from build123d import *

# Parameters (mm, degrees)
F0_R     = 25.4
F0_R_2   = 24.13
F1_DEPTH = 57.15
F3_DEPTH = 50.8


with BuildPart() as f1:
    # F0 (on Right) → F1 (new body, symmetric)
    with BuildSketch(Plane.YZ):
        with Locations((0, -25.4)):
            Circle(F0_R)
        with Locations((0, -25.4)):
            Circle(F0_R_2, mode=Mode.SUBTRACT)
    extrude(amount=F1_DEPTH, both=True)

    # F2 (on Top) → F3 (cut)
    with BuildSketch(Plane.XY):
        with BuildLine():
            ThreePointArc((48.895, -19.05), (47.9650640303, -16.8049359697), (45.72, -15.875))
            ThreePointArc((45.72, -15.875), (43.4749359697, -21.2950640303), (48.895, -19.05))
        make_face()
        with BuildLine():
            ThreePointArc((-42.545, -19.05), (-43.4749359697, -16.8049359697), (-45.72, -15.875))
            ThreePointArc((-45.72, -15.875), (-47.9650640303, -21.2950640303), (-42.545, -19.05))
        make_face()
    extrude(amount=-F3_DEPTH, mode=Mode.SUBTRACT)


solid = f1.part
Work out the finished part from the listing and answer in its coordinate system (mm). Coordinates: 2 decimals unless noted, no trailing zeros. Order: outer loops, then holes, each group sorted by start corner. A loop starts at its lowest first (then second) coordinate and runs counter-clockwise, first axis right, second up. Notation, with made-up numbers: (89.5, 44) - (110.5, 44) arc R10 cw to (110.5, 59) - close; hole circle Ø7 at (5, -35). An arc over 180 degrees is marked (long way). Put each result on its own line as item: value. Start each with the question number.
1) Flat-ended cylindrical pins translate along their axes: pin 1 (10 mm diameter, centred on x = -45.72, y = -19.05, fed in from -Z); pin 2 (2 mm diameter, centred on x = -20, z = -13.5, fed in from -Y); pin 3 (1.5 mm diameter, centred on x = -26.5, y = 10, fed in from +Z). Find the tip coordinate at first contact, or state that the pin passes through.
2) Find the intervals of material crossed by line 1 (X direction, y = -19, z = -9); line 2 (Z direction, x = 39.5, y = -1); line 3 (Z direction, x = -42, y = -9.5), in increasing order. Write a range as from..to.
3) For a pull along Y with two mould halves and no side action, classify faces 1 (the cylindrical face through (0.8, -20.157, -40.856)), 2 (the flat face through (57.15, 22.5, -34.7)), 3 (the cylindrical face through (-0.8, 23.016, -18.152)) as released by +Y, released by -Y, zero draft, split by the parting line, or undercut.
4) Find section A-A (y = 0). Give the vertices of the cut face in (x, z), plus the area to 3 significant figures.
5) Find section C-C (x = -35.5). Give the vertices of the cut face in (y, z), plus the area to 3 significant figures.
6) Find section B-B (x = -47). Give the vertices of the cut face in (y, z).
Results list:
1. pin 1: stops at z = -46.56
1. pin 2: stops at y = -22.94
1. pin 3: stops at z = -1.74
2. line 1: x = -57.15..-48.89, -42.55..42.55, 48.89..57.15
2. line 2: z = -50.78..-49.51, -1.29..-0.02
2. line 3: z = -48.96..-47.58, -3.22..-1.84
3. face 1: split by the parting line
3. face 2: zero draft
3. face 3: undercut
4. outline: (-57.15, -50.8) - (57.15, -50.8) - (57.15, -49.53) - (-57.15, -49.53) - close; (-57.15, -1.27) - (57.15, -1.27) - (57.15, 0) - (-57.15, 0) - close
4. area: 290 mm^2
5. outline: circle Ø50.8 at (0, -25.4); hole circle Ø48.26 at (0, -25.4)
5. area: 198 mm^2
6. outline: (-21.96, -38.17) - (-21.96, -35.41) arc R24.13 cw to (-21.96, -15.39) - (-21.96, -12.63) arc R25.4 ccw to start; (-16.14, -45.01) arc R25.4 ccw (long way) to (-16.14, -5.79) - (-16.14, -7.47) arc R24.13 cw (long way) to (-16.14, -43.33) - close
